CAD build for the part. Positions are in the model's coordinates, mm. Face numbers are marked on the shaded views. A direction names the side the tool comes from. Give positions to 0.01 mm unless a question says otherwise; leave off trailing zeros. Loops run counter-clockwise (first coordinate to the right, second up) from the corner with the lowest first, then second, coordinate; pieces in that order, holes last.
Item 1: Saw through at D-D on z = -9.5. Give the cut face in (x, y).
Item 2: Saw through at C-C on x = 29.5. Give the cut face in (y, z).
Item 3: Saw through at A-A on z = 17. Give the cut face in (x, y).
Item 4: Which spindle directions (+Z, -Z, +X, -X, +Y, -Y) get a long thin tool onto all of the face, cutting with end or side? Do the marked faces 1 and 2. Say none if no direction does.
Item 5: Saw through at B-B on y = 4. Give the cut face in (x, z).
Item 6: Drop flat-ended pins along their axis: P1, Ø5, axis at x = 25, z = 0.5, coming from the -Y side; P2, Ø1, axis at y = 21, z = 6, coming from the +X side; P3, Ø2.5, axis at y = 4, z = -17, coming from the -X side; P4, Ø5, axis at y = 4, z = 17, coming from the -X side. Give the stop position or say it passes through.
Item 7: Probe probe 1 along Y at (x, z) = (15.5, 17); probe 2 along Z at (x, y) = (16, 39); probe 3 along X at (y, z) = (23.5, -17). List the from-to ranges inside material, lowest first.
from build123d import *

# Parameters (mm, degrees)
SKETCH1_W           = 34
SKETCH1_H           = 42
BOSS_EXTRUDE1_DEPTH = 42
SKETCH2_R           = 11
BOSS_EXTRUDE2_DEPTH = 2
SKETCH3_R           = 2.5
BOSS_EXTRUDE3_DEPTH = 2
BOSS_EXTRUDE4_DEPTH = 15
CHAMFER1_SIZE       = 3
SKETCH5_R           = 1.5
CUT_EXTRUDE1_DEPTH  = 2


with BuildPart() as part:
    # Sketch1 → Boss-Extrude1 (new body)
    with BuildSketch(Plane(origin=(0, 0, 0), x_dir=(1, 0, 0), z_dir=(0, 1, 0))):
        Rectangle(SKETCH1_W, SKETCH1_H)
    extrude(amount=BOSS_EXTRUDE1_DEPTH)

    # Sketch2 → Boss-Extrude2 (add)
    with BuildSketch(Plane(origin=(17, 0, 0), x_dir=(0, 0, -1), z_dir=(1, 0, 0))):
        with Locations((0, 21)):
            Circle(SKETCH2_R)
    extrude(amount=BOSS_EXTRUDE2_DEPTH)

    # Sketch3 → Boss-Extrude3 (add)
    with BuildSketch(Plane(origin=(19, 0, 0), x_dir=(0, 0, -1), z_dir=(1, 0, 0))):
        with Locations((0, 21)):
            Circle(SKETCH3_R)
    extrude(amount=BOSS_EXTRUDE3_DEPTH)

    # Sketch4 → Boss-Extrude4 (add)
    with BuildSketch(Plane(origin=(21, 0, 0), x_dir=(0, 0, -1), z_dir=(1, 0, 0))):
        with BuildLine():
            Line((1.5, 23), (-1.5, 23))
            ThreePointArc((-1.5, 23), (0, 18.5), (1.5, 23))
        make_face()
    extrude(amount=BOSS_EXTRUDE4_DEPTH)

    # Chamfer1
    chamfer1_edges = [part.edges().sort_by_distance(p)[0] for p in [
        (0, 42, -21),
        (0, 0, -21),
        (0, 0, 21),
        (0, 42, 21),
    ]]
    chamfer(chamfer1_edges, length=CHAMFER1_SIZE)

    # Sketch5 → Cut-Extrude1 (cut)
    with BuildSketch(Plane(origin=(17, 0, 0), x_dir=(0, 0, -1), z_dir=(1, 0, 0))):
        with Locations((-17, 38)):
            Circle(SKETCH5_R)
        with Locations((-17, 4)):
            Circle(SKETCH5_R)
        with Locations((17, 4)):
            Circle(SKETCH5_R)
        with Locations((17, 38)):
            Circle(SKETCH5_R)
    cut_extrude1 = extrude(amount=-CUT_EXTRUDE1_DEPTH, mode=Mode.SUBTRACT)

    # Mirror1: Cut-Extrude1 across plane
    add(cut_extrude1.mirror(Plane(origin=(0, 0, 0), x_dir=(0, 0, 1), z_dir=(1, 0, 0))), mode=Mode.SUBTRACT)


solid = part.part
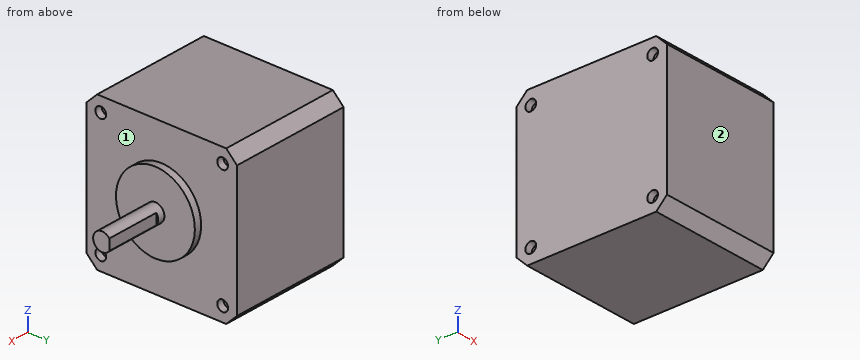
Results below:
1. outline: (-17, 0) - (17, 0) - (17, 15.45) - (19, 15.45) - (19, 26.55) - (17, 26.55) - (17, 42) - (-17, 42) - close
2. outline: (23, -1.5) - (23, 1.5) arc R2.5 ccw (long way) to start
3. outline: (-17, 0) - (17, 0) - (17, 2.5) - (15, 2.5) - (15, 5.5) - (17, 5.5) - (17, 36.5) - (15, 36.5) - (15, 39.5) - (17, 39.5) - (17, 42) - (-17, 42) - (-17, 39.5) - (-15, 39.5) - (-15, 36.5) - (-17, 36.5) - (-17, 5.5) - (-15, 5.5) - (-15, 2.5) - (-17, 2.5) - close
4. face 1: +X
4. face 2: +Z, -Z, +X, -X, -Y
5. outline: (-17, -21) - (17, -21) - (17, -18.5) - (15, -18.5) - (15, -15.5) - (17, -15.5) - (17, 15.5) - (15, 15.5) - (15, 18.5) - (17, 18.5) - (17, 21) - (-17, 21) - (-17, 18.5) - (-15, 18.5) - (-15, 15.5) - (-17, 15.5) - (-17, -15.5) - (-15, -15.5) - (-15, -18.5) - (-17, -18.5) - close
6. P1: stops at y = 18.5
6. P2: stops at x = 19
6. P3: stops at x = -15
6. P4: stops at x = -17
7. probe 1: y = 0 to 2.5, 5.5 to 36.5, 39.5 to 42
7. probe 2: z = -21 to -18.12, -15.88 to 15.88, 18.12 to 21
7. probe 3: x = -17 to 17
